Part model, mm, in its own coordinate system. A direction names the side the tool comes from. Coordinates: 2 decimals unless noted, no trailing zeros. Order: outer loops, then holes, each group sorted by start corner. A loop starts at its lowest first (then second) coordinate and runs counter-clockwise, first axis right, second up.
1) Mould opens along Z. For faces 4 (the flat face through (14, -16, 25.4)), 5 (the flat face through (4, -9, 0)), 6 (the flat face through (4, 19.818, 13)) say: +Z half, -Z half, draft (parallel to the pull), parting line (faces both ways), or undercut.
2) Cut at C-C (z = 30). List the corners of the cut face in (x, y), and give its area (3 significant figures).
3) Cut at B-B (y = -6.5). List the corners of the cut face in (x, z).
4) Cut at D-D (y = -16). List the corners of the cut face in (x, z), and give its area (3 significant figures).
5) Cut at A-A (x = 39). List the corners of the cut face in (y, z).
6) Wall check: L1, parallel to Z at x = 35, y = -32.5; L2, parallel to Z at x = 14, y = -14.5; L3, parallel to Y at x = -1, z = 27. Give the ranges that are in metal, low to high.
7) Tool access for faces 1 (the flat face through (1.59, 2.21, 31.46)), 2 (the flat face through (1.553, -11.119, 31.315)), 3 (the cylindrical face through (-12.4, -7.8, 29.7)): list every direction of +Z, -Z, +X, -X, +Y, -Y with a clear straight run to the whole face (end or side of a thin tool).
8) Pin check, flat tips, straight feed: pin 1 Ø1 at (y, z) = (-18, 32) entering from -X; pin 2 Ø1.5 at (x, z) = (-10.5, 29) entering from +Y; pin 3 Ø2 at (x, z) = (18.5, 26.5) entering from -Y; pin 4 Ø4 at (x, z) = (3, 32) entering from -Y. Stop position of each tip, or through.
```python
from build123d import *

# Parameters (mm, degrees)
F0_W     = 90.149514
F0_H     = 58.809195
F1_DEPTH = 25.4
F2_R     = 14.165363
F3_DEPTH = 38.1
F5_DEPTH = 261.366
F7_DEPTH = 25.4


with BuildPart() as f1:
    # F0 (on Top) → F1 (new body)
    with BuildSketch(Plane.XY):
        with Locations((4.97758, -9.586451)):
            Rectangle(F0_W, F0_H)
    extrude(amount=F1_DEPTH)

    # F2 (on Top) → F3 (join)
    with BuildSketch(Plane.XY):
        with Locations((1.751372, -8.388145)):
            Circle(F2_R)
    extrude(amount=F3_DEPTH)

    # F4 (on Front) → F5 (cut)
    with BuildSketch(Plane.XZ):
        Polygon((15.946694, 45.627825), (-27.192339, 42.125084), (15.946694, 25.901856), align=None)
    extrude(amount=F5_DEPTH, mode=Mode.SUBTRACT)

    # F6 (on Front) → F7 (cut)
    with BuildSketch(Plane.XZ):
        Polygon((-12.628307, 43.968629), (-12.443951, 36.963146), (15.76234, 25.901856), (15.76234, 43.968629), align=None)
    extrude(amount=-F7_DEPTH, mode=Mode.SUBTRACT)


solid = f1.part
```
Geometry check:
1. face 4: +Z half
1. face 5: -Z half
1. face 6: draft
2. outline: (5.05, -22.16) - (5.05, 0) - (5.31, 0) - (5.31, 5.32) arc R14.17 ccw (long way) to start
2. area: 409 mm2
3. outline: (-40.1, 0) - (50.05, 0) - (50.05, 25.4) - (15.79, 25.4) - (15.79, 25.96) - (-12.29, 36.52) - (-12.29, 25.4) - (-40.1, 25.4) - close
4. outline: (-40.1, 0) - (50.05, 0) - (50.05, 25.4) - (13.7, 25.4) - (13.7, 26.75) - (-10.2, 35.73) - (-10.2, 25.4) - (-40.1, 25.4) - close
4. area: 2,430 mm2
5. outline: (-38.99, 0) - (19.82, 0) - (19.82, 25.4) - (-38.99, 25.4) - close
6. L1: z = 0 to 25.4
6. L2: z = 0 to 26.63
6. L3: y = -22.28 to 5.51
7. face 1: +Z, +X, +Y, -Y
7. face 2: +Z, +X, -Y
7. face 3: +Z
8. pin 1: stops at x = -9.09
8. pin 2: stops at y = -0.12
8. pin 3: passes through
8. pin 4: stops at y = -22.55
